Read the model definition and answer for the solid it produces. Units are mm, in the model's axes. A direction names the side the tool comes from. Round coordinates to 2 decimals unless told otherwise and drop trailing zeros. Write each loop counter-clockwise with the first axis right and the second up, starting at its lowest first coordinate (ties: lowest second). Pieces come first, ordered by that corner, then holes. Notation, with made-up numbers: (-16, 1.25) - (31, 1.25) arc R18 ccw to (31, 33.25) - close; hole circle Ø7 at (51, 24.25). An arc over 180 degrees is marked (long way). Answer as CSV lines item,"result". Start each with the question number.
1) Find section C-C on x = 3. Determine the outline of the cut face in (y, z), then the cut area to 3 significant figures.
2) Find section B-B on y = -0.4. Determine the outline of the cut face in (x, z).
3) Each of these flat-tipped pins is pushed along its axis until it touches: pin 1 (2.5 mm diameter, centred on x = -3, z = -7.7, fed in from +Y); pin 2 (1.2 mm diameter, centred on x = 3, z = -7.7, fed in from -Y); pin 3 (0.5 mm diameter, centred on y = -0.5, z = -7, fed in from -X). Where does it stop, or does it pass through?
4) Which of the six approach directions +Z, -Z, +X, -X, +Y, -Y give full straight-line access (tool end or side, diameter ignored) to faces 1 (the flat face through (1, -0.5, -8.4)), 2 (the flat face through (-6, -0.5, -6.9)), 3 (the cylindrical face through (-4, -0.5, -7.7))?
5) Consider line 1 along Z through (x, y) = (3, -0.7); line 2 along X through (y, z) = (-0.2, -7); line 3 along X through (y, z) = (-0.75, -8.5). Determine where each line is inside the solid, lowest interval first.
6) Find section A-A on z = 1.5. Determine the outline of the cut face in (x, y).
7) For a pull along X with two mould halves and no side action, classify faces 4 (the flat face through (6, -0.5, -7)), 5 (the flat face through (-1, -0.5, -8.5)), 6 (the cylindrical face through (-3.41, -0.49, -9.4)) as +X half, -X half, draft (parallel to the pull), parting line (faces both ways), or undercut.
8) Find section D-D on z = -7.7. Determine the outline of the cut face in (x, y).
from build123d import *

# Parameters (mm, degrees)
F0_R     = 1
F1_DEPTH = 1


with BuildPart() as f1:
    # F0 (on Front) → F1 (new body)
    with BuildSketch(Plane.XZ):
        with BuildLine():
            ThreePointArc((-1, -6.928203), (-6.982028, 0.501287), (0, 7))
            Line((0, 7), (0, 8.5))
            ThreePointArc((0, 8.5), (-7.781249, 3.420841), (-6.263158, -5.746551))
            ThreePointArc((-6.263158, -5.746551), (-6.068109, -6.059878), (-6, -6.422616))
            Line((-6, -6.422616), (-6, -7.483315))
            ThreePointArc((-6, -7.483315), (-5.881917, -7.954719), (-5.555556, -8.314794))
            ThreePointArc((-5.555556, -8.314794), (-3.378195, -9.412109), (-1, -9.949874))
            Line((-1, -9.949874), (-1, -6.928203))
        make_face()
        with Locations((-3, -7.7)):
            Circle(F0_R, mode=Mode.SUBTRACT)
        with BuildLine():
            ThreePointArc((0, 7), (6.982028, 0.501287), (1, -6.928203))
            Line((1, -6.928203), (1, -9.949874))
            ThreePointArc((1, -9.949874), (3.378195, -9.412109), (5.555556, -8.314794))
            ThreePointArc((5.555556, -8.314794), (5.881917, -7.954719), (6, -7.483315))
            Line((6, -7.483315), (6, -6.422616))
            ThreePointArc((6, -6.422616), (6.068109, -6.059878), (6.263158, -5.746551))
            ThreePointArc((6.263158, -5.746551), (7.781249, 3.420841), (0, 8.5))
            Line((0, 8.5), (0, 7))
        make_face()
        with Locations((3, -7.7)):
            Circle(F0_R, mode=Mode.SUBTRACT)
    extrude(amount=F1_DEPTH)


solid = f1.part
Check values:
1,outline,"(-1, -9.54) - (0, -9.54) - (0, -8.7) - (-1, -8.7) - close; (-1, -6.7) - (0, -6.7) - (0, -6.32) - (-1, -6.32) - close; (-1, 6.32) - (0, 6.32) - (0, 7.95) - (-1, 7.95) - close"
1,area,"2.84 mm^2"
2,outline,"(-6.26, -5.75) arc R1 cw to (-6, -6.42) - (-6, -7.48) arc R1 ccw to (-5.56, -8.31) arc R10 ccw to (-1, -9.95) - (-1, -6.93) arc R7 cw (long way) to (1, -6.93) - (1, -9.95) arc R10 ccw to (5.56, -8.31) arc R1 ccw to (6, -7.48) - (6, -6.42) arc R1 cw to (6.26, -5.75) arc R8.5 ccw to (0, 8.5) arc R8.5 ccw to start; hole circle Ø2 at (-3, -7.7); hole circle Ø2 at (3, -7.7)"
3,pin 1,"stops at y = 0"
3,pin 2,"passes through"
3,pin 3,"stops at x = -6"
4,face 1,"-Z, +Y, -Y"
4,face 2,"-Z, -X, +Y, -Y"
4,face 3,"+Y, -Y"
5,line 1,"z = -9.54 to -8.7, -6.7 to -6.32, 6.32 to 7.95"
5,line 2,"x = -6 to -3.71, -2.29 to -1, 1 to 2.29, 3.71 to 6"
5,line 3,"x = -5.27 to -3.6, -2.4 to -1, 1 to 2.4, 3.6 to 5.27"
6,outline,"(-8.37, -1) - (-6.84, -1) - (-6.84, 0) - (-8.37, 0) - close; (6.84, -1) - (8.37, -1) - (8.37, 0) - (6.84, 0) - close"
7,face 4,"+X half"
7,face 5,"undercut"
7,face 6,"-X half"
8,outline,"(-5.98, -1) - (-4, -1) - (-4, 0) - (-5.98, 0) - close; (-2, -1) - (-1, -1) - (-1, 0) - (-2, 0) - close; (1, -1) - (2, -1) - (2, 0) - (1, 0) - close; (4, -1) - (5.98, -1) - (5.98, 0) - (4, 0) - close"
